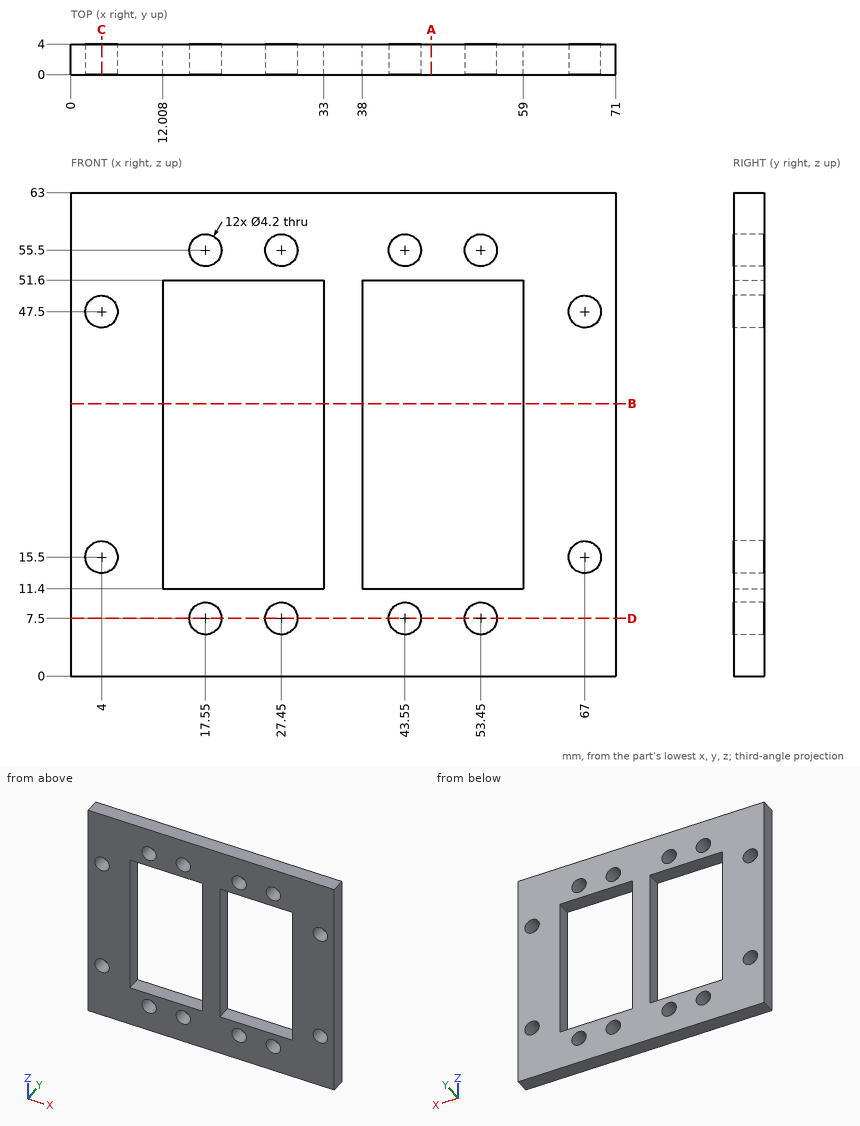
Print and shaded views of the part. All mm, measured from the part's lowest x, y and z. Round coordinates to 2 decimals unless told otherwise and drop trailing zeros. Write each loop counter-clockwise with the first axis right and the second up, starting at its lowest first coordinate (ties: lowest second). Pieces come first, ordered by that corner, then holes.
(1) Slice it at B-B, the plane z = 35.5. Write the cut outline in (x, y).
(2) Slice it at A-A, the plane x = 47. Write the cut outline in (y, z), and give its area (3 significant figures).
(3) Slice it at D-D, the plane z = 7.5. Write the cut outline in (x, y), and give its area (3 significant figures).
(4) Drop a flat-ended pin along its axis: P1, Ø3.5, axis at x = 4, z = 15.5, coming from the -Y side. Give the stop position or say it passes through.
(5) Probe line 1 along X through (y, z) = (2.95, 47.5); line 2 along Z through (x, y) = (43.55, 2.55); line 3 along X through (y, z) = (0.5, 27). List the from-to ranges inside material, lowest first.
(6) Slice it at C-C, the plane x = 4. Write the cut outline in (y, z), and give its area (3 significant figures).
From the geometry:
1. outline: (0, 0) - (12.01, 0) - (12.01, 4) - (0, 4) - close; (33, 0) - (38, 0) - (38, 4) - (33, 4) - close; (59, 0) - (71, 0) - (71, 4) - (59, 4) - close
2. outline: (0, 0) - (4, 0) - (4, 11.4) - (0, 11.4) - close; (0, 51.6) - (4, 51.6) - (4, 63) - (0, 63) - close
2. area: 91.2 mm2
3. outline: (0, 0) - (15.45, 0) - (15.45, 4) - (0, 4) - close; (19.65, 0) - (25.35, 0) - (25.35, 4) - (19.65, 4) - close; (29.55, 0) - (41.45, 0) - (41.45, 4) - (29.55, 4) - close; (45.65, 0) - (51.35, 0) - (51.35, 4) - (45.65, 4) - close; (55.55, 0) - (71, 0) - (71, 4) - (55.55, 4) - close
3. area: 217 mm2
4. P1: passes through
5. line 1: x = 0 to 1.9, 6.1 to 12.01, 33 to 38, 59 to 64.9, 69.1 to 71
5. line 2: z = 0 to 5.4, 9.6 to 11.4, 51.6 to 53.4, 57.6 to 63
5. line 3: x = 0 to 12.01, 33 to 38, 59 to 71
6. outline: (0, 0) - (4, 0) - (4, 13.4) - (0, 13.4) - close; (0, 17.6) - (4, 17.6) - (4, 45.4) - (0, 45.4) - close; (0, 49.6) - (4, 49.6) - (4, 63) - (0, 63) - close
6. area: 218 mm2
